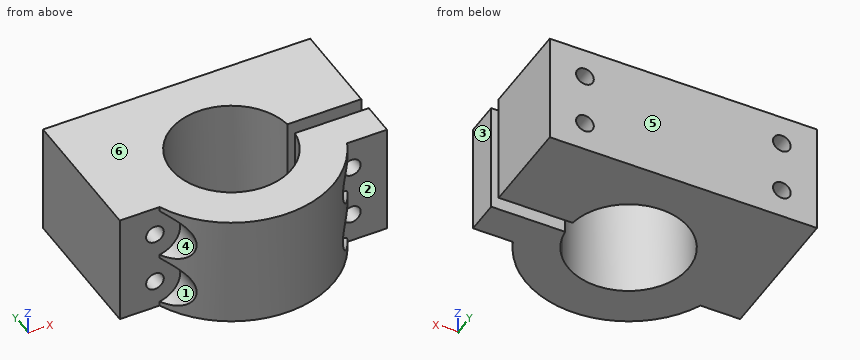
```python
from build123d import *

# Parameters (mm, degrees)
F1_DEPTH = 40
F2_R     = 3.15
F3_DEPTH = 72.801
F4_START = -51
F2_R_2   = 9
F4_DEPTH = 21.8010001


with BuildPart() as f1:
    # F0 (on Top) → F1 (new body)
    with BuildSketch(Plane.XY):
        with BuildLine():
            Line((-47.5, -25.5), (-33.3436650655, -25.5))
            ThreePointArc((-33.3436650655, -25.5), (-30.4663749074, 9.0188353073), (0, 25.5))
            Line((0, 25.5), (-47.5, 25.5))
            Line((-47.5, 25.5), (-47.5, -25.5))
        make_face()
        with BuildLine():
            Line((36.3140468689, -8.4), (47.5, -8.4))
            Line((47.5, -8.4), (47.5, 25.5))
            Line((47.5, 25.5), (0, 25.5))
            ThreePointArc((0, 25.5), (24.8390821086, 15.7078935656), (36.3140468689, -8.4))
        make_face()
        with BuildLine():
            ThreePointArc((0, 25.5), (-30.4663749074, 9.0188353073), (-33.3436650655, -25.5))
            Line((-33.3436650655, -25.5), (-15.6460857725, -25.5))
            ThreePointArc((-15.6460857725, -25.5), (-8.9979547856, 8.5164056838), (21.2534703049, -8.4))
            Line((21.2534703049, -8.4), (36.3140468689, -8.4))
            ThreePointArc((36.3140468689, -8.4), (24.8390821086, 15.7078935656), (0, 25.5))
        make_face()
        with BuildLine():
            Line((15.6460857725, -25.5), (33.3436650655, -25.5))
            ThreePointArc((33.3436650655, -25.5), (35.3504131233, -19.5780350319), (36.3140468689, -13.4))
            Line((36.3140468689, -13.4), (21.2534703049, -13.4))
            ThreePointArc((21.2534703049, -13.4), (19.4164056838, -19.8979547856), (15.6460857725, -25.5))
        make_face()
        with BuildLine():
            ThreePointArc((-33.3436650655, -25.5), (0, -47.3), (33.3436650655, -25.5))
            Line((33.3436650655, -25.5), (15.6460857725, -25.5))
            ThreePointArc((15.6460857725, -25.5), (0, -32.3), (-15.6460857725, -25.5))
            Line((-15.6460857725, -25.5), (-33.3436650655, -25.5))
        make_face()
        with BuildLine():
            Line((33.3436650655, -25.5), (47.5, -25.5))
            Line((47.5, -25.5), (47.5, -13.4))
            Line((47.5, -13.4), (36.3140468689, -13.4))
            ThreePointArc((36.3140468689, -13.4), (35.3504131233, -19.5780350319), (33.3436650655, -25.5))
        make_face()
    extrude(amount=F1_DEPTH)

    # F2 (on face) → F3 (cut, through all)
    with BuildSketch(Plane(origin=(0, 25.5, 0), x_dir=(-1, 0, 0), z_dir=(0, 1, 0))):
        with Locations((-35, 29.5)):
            Circle(F2_R)
        with Locations((-35, 10.5)):
            Circle(F2_R)
        with Locations((35, 29.5)):
            Circle(F2_R)
        with Locations((35, 10.5)):
            Circle(F2_R)
    extrude(amount=-F3_DEPTH, mode=Mode.SUBTRACT)

    # F2 (on face) → F4 (cut)
    with BuildSketch(Plane(origin=(0, 25.5, 0), x_dir=(-1, 0, 0), z_dir=(0, 1, 0)).offset(F4_START)):
        with Locations((-35, 29.5)):
            Circle(F2_R_2)
        with Locations((-35, 29.5)):
            Circle(F2_R, mode=Mode.SUBTRACT)
        with Locations((-35, 10.5)):
            Circle(F2_R_2)
        with Locations((-35, 10.5)):
            Circle(F2_R, mode=Mode.SUBTRACT)
        with Locations((35, 10.5)):
            Circle(F2_R_2)
        with Locations((35, 10.5)):
            Circle(F2_R, mode=Mode.SUBTRACT)
        with Locations((35, 29.5)):
            Circle(F2_R_2)
        with Locations((35, 29.5)):
            Circle(F2_R, mode=Mode.SUBTRACT)
    extrude(amount=-F4_DEPTH, mode=Mode.SUBTRACT)


solid = f1.part
```
The model under review builds one solid part; all positions refer to its coordinate system, in mm. Face numbers are marked on the shaded views. A direction names the side the tool comes from. Give positions to 0.01 mm unless a question says otherwise; leave off trailing zeros. Write each loop counter-clockwise with the first axis right and the second up, starting at its lowest first coordinate (ties: lowest second). Pieces come first, ordered by that corner, then holes.
(1) Consider section D-D, the plane x = -35. Give the boundary of the cut face in (y, z), and give its area (3 significant figures).
(2) Consider section A-A, the plane z = 29.5. Give the boundary of the cut face in (x, y), and give its area (3 significant figures).
(3) The part is to be moulded in two halves that separate along Z. For the marked faces 4, 5 and 6, say which applies: released by +Z, released by -Z, zero draft, split by the parting line, or undercut.
(4) Consider section C-C, the plane y = -10.9. Give the boundary of the cut face in (x, z).
(5) For P1, Ø6, axis at x = 13.5, z = 16.5, coming from the -Y side; P2, Ø7, axis at x = 35, z = 10.5, coming from the -Y side; P3, Ø11, axis at x = 34, z = 19, coming from the -Y side, all flat-tipped, find the tip position at first contact; note any pin that passes through.
(6) To check wall thickness, follow L1, parallel to Z at x = 35, y = 13; L2, parallel to X at y = -16, z = 10; L3, parallel to X at y = -8, z = 28.5. State the ranges of each line that lie inside material, in increasing order.
(7) Tool access review of the marked faces 1, 2 and 3: name each direction out of +Z, -Z, +X, -X, +Y, -Y from which nothing blocks a thin tool from reaching the whole face with its end or side.
(8) Consider section B-B, the plane x = 0. Give the boundary of the cut face in (y, z).
Returned:
1. outline: (-25.5, 0) - (25.5, 0) - (25.5, 7.35) - (-25.5, 7.35) - close; (-25.5, 13.65) - (25.5, 13.65) - (25.5, 26.35) - (-25.5, 26.35) - close; (-25.5, 32.65) - (25.5, 32.65) - (25.5, 40) - (-25.5, 40) - close
1. area: 1,400 mm2
2. outline: (-47.5, -25.5) - (-38.15, -25.5) - (-38.15, 25.5) - (-47.5, 25.5) - close; (-31.85, -25.5) - (-26, -25.5) - (-26, -36.37) arc R36.4 ccw to (26, -36.37) - (26, -25.5) - (31.85, -25.5) - (31.85, -13.4) - (21.25, -13.4) arc R21.4 cw (long way) to (21.25, -8.4) - (31.85, -8.4) - (31.85, 25.5) - (-31.85, 25.5) - close; (38.15, -25.5) - (47.5, -25.5) - (47.5, -13.4) - (38.15, -13.4) - close; (38.15, -8.4) - (47.5, -8.4) - (47.5, 25.5) - (38.15, 25.5) - close
2. area: 3,620 mm2
3. face 4: undercut
3. face 5: zero draft
3. face 6: released by +Z
4. outline: (-47.5, 0) - (-21.4, 0) - (-21.4, 40) - (-47.5, 40) - close; hole circle Ø6.3 at (-35, 10.5); hole circle Ø6.3 at (-35, 29.5)
5. P1: stops at y = -45.75
5. P2: stops at y = -25.5
5. P3: stops at y = -33.54
6. L1: z = 0 to 7.35, 13.65 to 26.35, 32.65 to 40
6. L2: x = -47.5 to -38.11, -31.89 to -20.78, 20.78 to 31.89, 38.11 to 47.5
6. L3: x = -47.5 to -37.99, -32.01 to -21.2, 21.2 to 32.01, 37.99 to 47.5
7. face 1: -X, -Y
7. face 2: +X, -Y
7. face 3: +Z, -Z, +X, +Y, -Y
8. outline: (-47.3, 0) - (-32.3, 0) - (-32.3, 40) - (-47.3, 40) - close; (10.5, 0) - (25.5, 0) - (25.5, 40) - (10.5, 40) - close
